```python
from build123d import *

# Parameters (mm, degrees)
SKETCH2_W           = 18
SKETCH2_H           = 12
BOSS_EXTRUDE1_DEPTH = 1
FILLET1_R           = 1
SKETCH3_W           = 18
SKETCH3_H           = 6
BOSS_EXTRUDE2_DEPTH = 1
SKETCH4_W           = 2
SKETCH4_H           = 6
BOSS_EXTRUDE3_DEPTH = 1
FILLET2_START       = -4
FILLET2_DEPTH       = 8
FILLET2_START_2     = -3
FILLET2_2_DEPTH     = 6


with BuildPart() as part:
    # Sketch2 → Boss-Extrude1 (new body)
    with BuildSketch(Plane(origin=(0, 0, 0), x_dir=(1, 0, 0), z_dir=(0, 1, 0))):
        Rectangle(SKETCH2_W, SKETCH2_H)
    extrude(amount=BOSS_EXTRUDE1_DEPTH)

    # Fillet1
    fillet1_edges = [part.edges().sort_by_distance(p)[0] for p in [
        (9, 0.5, 6),
        (-9, 0.5, 6),
        (-9, 0.5, -6),
        (9, 0.5, -6),
    ]]
    fillet(fillet1_edges, radius=FILLET1_R)

    # Sketch3 → Boss-Extrude2 (add)
    with BuildSketch(Plane(origin=(0, 1, 0), x_dir=(1, 0, 0), z_dir=(0, 1, 0))):
        Rectangle(SKETCH3_W, SKETCH3_H)
    extrude(amount=BOSS_EXTRUDE2_DEPTH)

    # Sketch4 → Boss-Extrude3 (add)
    with BuildSketch(Plane(origin=(0, 2, 0), x_dir=(1, 0, 0), z_dir=(0, 1, 0))):
        Rectangle(SKETCH4_W, SKETCH4_H)
        with Locations((-4, 0)):
            Rectangle(SKETCH4_W, SKETCH4_H)
        with Locations((4, 0)):
            Rectangle(SKETCH4_W, SKETCH4_H)
    extrude(amount=BOSS_EXTRUDE3_DEPTH)

    # Fillet2: read off the stored shape, not the designer's step
    # Fillet2 outline → Fillet2 (cut)
    with BuildSketch(Plane.XY.offset(FILLET2_START)):
        with BuildLine():
            ThreePointArc((-5, 2.5), (-4.853553391, 2.853553391), (-4.5, 3))
            Line((-4.5, 3), (-5, 3))
            Line((-5, 3), (-5, 2.5))
        make_face()
        with BuildLine():
            ThreePointArc((-3.5, 3), (-3.146446609, 2.853553391), (-3, 2.5))
            Line((-3, 2.5), (-3, 3))
            Line((-3, 3), (-3.5, 3))
        make_face()
        with BuildLine():
            ThreePointArc((-1, 2.5), (-0.853553391, 2.853553391), (-0.5, 3))
            Line((-0.5, 3), (-1, 3))
            Line((-1, 3), (-1, 2.5))
        make_face()
        with BuildLine():
            ThreePointArc((0.5, 3), (0.853553391, 2.853553391), (1, 2.5))
            Line((1, 2.5), (1, 3))
            Line((1, 3), (0.5, 3))
        make_face()
        with BuildLine():
            ThreePointArc((3, 2.5), (3.146446609, 2.853553391), (3.5, 3))
            Line((3.5, 3), (3, 3))
            Line((3, 3), (3, 2.5))
        make_face()
        with BuildLine():
            ThreePointArc((4.5, 3), (4.853553391, 2.853553391), (5, 2.5))
            Line((5, 2.5), (5, 3))
            Line((5, 3), (4.5, 3))
        make_face()
    extrude(amount=FILLET2_DEPTH, mode=Mode.SUBTRACT)

    # Fillet2 2 outline → Fillet2 2 (add)
    with BuildSketch(Plane.XY.offset(FILLET2_START_2)):
        with BuildLine():
            Line((-5, 2), (-5, 2.5))
            ThreePointArc((-5, 2.5), (-5.146446609, 2.146446609), (-5.5, 2))
            Line((-5.5, 2), (-5, 2))
        make_face()
        with BuildLine():
            Line((-3, 2), (-2.5, 2))
            ThreePointArc((-2.5, 2), (-2.853553391, 2.146446609), (-3, 2.5))
            Line((-3, 2.5), (-3, 2))
        make_face()
        with BuildLine():
            Line((-1, 2), (-1, 2.5))
            ThreePointArc((-1, 2.5), (-1.146446609, 2.146446609), (-1.5, 2))
            Line((-1.5, 2), (-1, 2))
        make_face()
        with BuildLine():
            Line((1, 2), (1.5, 2))
            ThreePointArc((1.5, 2), (1.146446609, 2.146446609), (1, 2.5))
            Line((1, 2.5), (1, 2))
        make_face()
        with BuildLine():
            Line((3, 2), (3, 2.5))
            ThreePointArc((3, 2.5), (2.853553391, 2.146446609), (2.5, 2))
            Line((2.5, 2), (3, 2))
        make_face()
        with BuildLine():
            ThreePointArc((5.5, 2), (5.146446609, 2.146446609), (5, 2.5))
            Line((5, 2.5), (5, 2))
            Line((5, 2), (5.5, 2))
        make_face()
    extrude(amount=FILLET2_2_DEPTH)


solid = part.part
```
Could you check a few things on this model? Use its own coordinates, in mm. A direction names the side the tool comes from. Round coordinates to 2 decimals unless told otherwise and drop trailing zeros. Write each loop counter-clockwise with the first axis right and the second up, starting at its lowest first coordinate (ties: lowest second). Pieces come first, ordered by that corner, then holes.
(1) Thinking about a two-plate mould opening in X: for faces 4 (the face through (-2, 2, 0)), 5 (the face through (2, 2, 0)), 6 (the face through (7, 2, 0)), 7 (the face through (8.699, 0.507, 5.715)), which applies, +X half, -X half, draft (parallel to the pull), parting line (faces both ways), or undercut?
Findings below:
face 4: undercut
face 5: undercut
face 6: draft
face 7: +X half
(2) Suppose I cut it at D-D on y = 1.4. Write out the boundary of the cut face in (x, z), and give its area (3 significant figures).
Findings below:
outline: (-9, -3) - (9, -3) - (9, 3) - (-9, 3) - close
area: 108 mm2
(3) Which directions (+Z, -Z, +X, -X, +Y, -Y) give clear straight access to the entire face, cutting with the end or side of a thin tool? Please do faces 1 (the face through (0, 1, -5)), 2 (the face through (0, 2, 3)), 3 (the face through (-7, 2, 0)).
Findings below:
face 1: -Z, +X, -X, +Y
face 2: +Z, +X, -X, +Y
face 3: +Z, -Z, -X, +Y
(4) Suppose I cut it at A-A on y = 2.25. Write out the boundary of the cut face in (x, z).
Findings below:
outline: (-5.07, -3) - (-2.93, -3) - (-2.93, 3) - (-5.07, 3) - close; (-1.07, -3) - (1.07, -3) - (1.07, 3) - (-1.07, 3) - close; (2.93, -3) - (5.07, -3) - (5.07, 3) - (2.93, 3) - close
(5) If I drill on probe 1 along X at (y, z) = (2.5, 1.25); probe 2 along X at (y, z) = (2.2, 0.25); probe 3 along Z at (x, y) = (7.5, 1.7), over which ranges is the centre line in solid material (lowest first)?
Findings below:
probe 1: x = -5 to -3, -1 to 1, 3 to 5
probe 2: x = -5.1 to -2.9, -1.1 to 1.1, 2.9 to 5.1
probe 3: z = -3 to 3
(6) For pin 1 (4 mm diameter, centred on x = 8, z = -0.5, fed in from +Y); pin 2 (2.5 mm diameter, centred on x = -4, z = 4.5, fed in from +Y), each with a flat end and sliding along its axis, tell me the tip position at first contact or that it passes through.
Findings below:
pin 1: stops at y = 2
pin 2: stops at y = 1
(7) Suppose I cut it at C-C on x = -6.25. Write out the boundary of the cut face in (y, z), and give its area (3 significant figures).
Findings below:
outline: (0, -6) - (1, -6) - (1, -3) - (2, -3) - (2, 3) - (1, 3) - (1, 6) - (0, 6) - close
area: 18.0 mm2
(8) Suppose I cut it at B-B on z = 1.25. Write out the boundary of the cut face in (x, y).
Findings below:
outline: (-9, 0) - (9, 0) - (9, 2) - (5.5, 2) arc R0.5 cw to (5, 2.5) arc R0.5 ccw to (4.5, 3) - (3.5, 3) arc R0.5 ccw to (3, 2.5) arc R0.5 cw to (2.5, 2) - (1.5, 2) arc R0.5 cw to (1, 2.5) arc R0.5 ccw to (0.5, 3) - (-0.5, 3) arc R0.5 ccw to (-1, 2.5) arc R0.5 cw to (-1.5, 2) - (-2.5, 2) arc R0.5 cw to (-3, 2.5) arc R0.5 ccw to (-3.5, 3) - (-4.5, 3) arc R0.5 ccw to (-5, 2.5) arc R0.5 cw to (-5.5, 2) - (-9, 2) - close
